```python
from build123d import *

# Parameters (mm, degrees)
F1_DEPTH = 10
F0_R     = 5
F2_DEPTH = 5
F0_W     = 12.0738212518
F0_H     = 31.9068175741
F3_DEPTH = 12.5
F4_R     = 5
F5_SIZE2 = 5
F5_SIZE  = 10
F7_DEPTH = 25
F8_W     = 7.5
F8_H     = 27.4257330972
F9_DEPTH = 15


with BuildPart() as f1:
    # F0 (on Front) → F1 (new body, symmetric)
    with BuildSketch(Plane.XZ):
        with BuildLine():
            Line((-21.1634319276, -26.7058201134), (-21.1634319276, -41.4115685539))
            ThreePointArc((-21.1634319276, -41.4115685539), (-10.6175206449, -34.455488704), (1.9829672237, -33.5438982608))
            Line((1.9829672237, -33.5438982608), (3.4650283433, -26.7058201134))
            Line((3.4650283433, -26.7058201134), (-8.6087929085, -26.7058201134))
            Line((-8.6087929085, -26.7058201134), (-21.1634319276, -26.7058201134))
        make_face()
    extrude(amount=F1_DEPTH, both=True)

    # F0 (on Front) → F2 (join, symmetric)
    with BuildSketch(Plane.XZ):
        with BuildLine():
            Line((-21.1634319276, -41.4115685539), (-21.1634319276, -53.1254634261))
            Line((-21.1634319276, -53.1254634261), (-19.8923903583, -53.1254634261))
            Line((-19.8923903583, -53.1254634261), (-11.2321363204, -53.1254634261))
            ThreePointArc((-11.2321363204, -53.1254634261), (-2.5718822826, -68.1254634261), (6.0883717553, -53.1254634261))
            Line((6.0883717553, -53.1254634261), (14.7486257931, -53.1254634261))
            Line((14.7486257931, -53.1254634261), (16.0196673624, -53.1254634261))
            Line((16.0196673624, -53.1254634261), (16.0196673624, -41.4115685539))
            ThreePointArc((16.0196673624, -41.4115685539), (9.6516199724, -36.3175292593), (1.9829672237, -33.5438982608))
            ThreePointArc((1.9829672237, -33.5438982608), (-10.6175206449, -34.455488704), (-21.1634319276, -41.4115685539))
        make_face()
        with Locations((-2.5718822826, -58.1254634261)):
            Circle(F0_R, mode=Mode.SUBTRACT)
        with BuildLine():
            Line((3.4650283433, -26.7058201134), (1.9829672237, -33.5438982608))
            ThreePointArc((1.9829672237, -33.5438982608), (9.6516199724, -36.3175292593), (16.0196673624, -41.4115685539))
            Line((16.0196673624, -41.4115685539), (16.0196673624, -26.7058201134))
            Line((16.0196673624, -26.7058201134), (3.4650283433, -26.7058201134))
        make_face()
    extrude(amount=F2_DEPTH, both=True)

    # F0 (on Front) → F3 (join, symmetric)
    with BuildSketch(Plane.XZ):
        with Locations((-2.5718822826, -10.7524113264)):
            Rectangle(F0_W, F0_H)
        Polygon((-4.447942134, 28.565781191), (-8.6087929085, 5.2009974606), (3.4650283433, 5.2009974606), (7.2547487569, 26.4817409097), align=None)
        Polygon((6.1142202467, 42.9687313735), (-4.447942134, 28.565781191), (7.2547487569, 26.4817409097), (16.6688518649, 39.3191555594), align=None)
    extrude(amount=F3_DEPTH, both=True)

    # F4
    f4_edges = [f1.edges().sort_by_distance(p)[0] for p in [
        (-8.608793, 0, 5.200997),
        (-4.447942, 0, 28.565781),
    ]]
    fillet(f4_edges, radius=F4_R)

    # F5
    f5_edges = [f1.edges().sort_by_distance(p)[0] for p in [
        (6.11422, 0, 42.968731),
    ]]
    f5_side = f1.faces().sort_by_distance((1.176582, 0, 36.235587))[0]
    chamfer(f5_edges, length=F5_SIZE, length2=F5_SIZE2, reference=f5_side)

    # F6 (on face) → F7 (cut)
    with BuildSketch(Plane(origin=(-15.3979489719, 0, 25.4772253764), x_dir=(0.8558343717, 0, 0.5172499669), z_dir=(-0.5172499669, 0, 0.8558343717))):
        with BuildLine():
            Line((30.657387603, 12.5), (30.657387603, 4.6880120664))
            ThreePointArc((30.657387603, 4.6880120664), (32.4777582205, 0), (30.657387603, -4.6880120664))
            Line((30.657387603, -4.6880120664), (30.657387603, -12.5))
            Line((30.657387603, -12.5), (39.1792431474, -12.5))
            Line((39.1792431474, -12.5), (39.1792431474, 12.5))
            Line((39.1792431474, 12.5), (30.657387603, 12.5))
        make_face()
        with BuildLine():
            Line((21.6556563973, 12.5), (21.6556563973, 9.3958744477))
            ThreePointArc((21.6556563973, 9.3958744477), (22.5944314954, 2.8906144363), (28.1230778906, 6.445016712))
            ThreePointArc((28.1230778906, 6.445016712), (29.4889605189, 5.7089196767), (30.657387603, 4.6880120664))
            Line((30.657387603, 4.6880120664), (30.657387603, 12.5))
            Line((30.657387603, 12.5), (21.6556563973, 12.5))
        make_face()
        with BuildLine():
            Line((30.657387603, -12.5), (30.657387603, -4.6880120664))
            ThreePointArc((30.657387603, -4.6880120664), (29.4889605189, -5.7089196767), (28.1230778906, -6.445016712))
            ThreePointArc((28.1230778906, -6.445016712), (22.5944314954, -2.8906144363), (21.6556563973, -9.3958744477))
            Line((21.6556563973, -9.3958744477), (21.6556563973, -12.5))
            Line((21.6556563973, -12.5), (30.657387603, -12.5))
        make_face()
    extrude(amount=-F7_DEPTH, mode=Mode.SUBTRACT)

    # F8 (on face) → F9 (cut)
    with BuildSketch(Plane(origin=(-21.1634319276, 0, 0), x_dir=(0, -1, 0), z_dir=(-1, 0, 0))):
        with Locations((0, -39.4125968775)):
            Rectangle(F8_W, F8_H)
    extrude(amount=-F9_DEPTH, mode=Mode.SUBTRACT)


solid = f1.part
```
Read the model definition and answer for the solid it produces. Units are mm, in the model's axes. A direction names the side the tool comes from. Coordinates: 2 decimals unless noted, no trailing zeros. Write each loop counter-clockwise with the first axis right and the second up, starting at its lowest first coordinate (ties: lowest second). Pieces come first, ordered by that corner, then holes. Notation, with made-up numbers: (19.5, 44) -> (63.5, 44) arc R3 cw to (63.5, 49) -> close; hole circle Ø11 at (-25.75, -3.5). An arc over 180 degrees is marked (long way). Return JSON: item names as keys, results as strings.
1. A cutting plane is placed at C-C (z = -29.5). Determine the outline of the cut face in (x, y).
Found:
{"outline": "(-21.16, -10) -> (2.86, -10) -> (2.86, -5) -> (16.02, -5) -> (16.02, 5) -> (2.86, 5) -> (2.86, 10) -> (-21.16, 10) -> (-21.16, 3.75) -> (-6.16, 3.75) -> (-6.16, -3.75) -> (-21.16, -3.75) -> close"}
2. A cutting plane is placed at D-D (x = -19). Determine the outline of the cut face in (y, z).
Found:
{"outline": "(-10, -39.28) -> (-5, -39.28) -> (-5, -53.13) -> (-3.75, -53.13) -> (-3.75, -26.71) -> (-10, -26.71) -> close; (3.75, -53.13) -> (5, -53.13) -> (5, -39.28) -> (10, -39.28) -> (10, -26.71) -> (3.75, -26.71) -> close"}
3. Determine the mould class of faces 1 (the face through (-12, 10, -31)), 2 (the face through (6.607, 2.937, 32.559)), 3 (the face through (-21.163, -6, -37)), 4 (the face through (-12, -10, -31)) for opening direction Y: pulls with the +Y half, pulls with the -Y half, needs draft (parallel to the pull), parting line crosses it, or undercut.
Found:
{"face 1": "pulls with the +Y half", "face 2": "undercut", "face 3": "needs draft", "face 4": "pulls with the -Y half"}
4. A cutting plane is placed at A-A (x = -14). Determine the outline of the cut face in (y, z).
Found:
{"outline": "(-10, -35.89) -> (-5, -35.89) -> (-5, -53.13) -> (-3.75, -53.13) -> (-3.75, -26.71) -> (-10, -26.71) -> close; (3.75, -53.13) -> (5, -53.13) -> (5, -35.89) -> (10, -35.89) -> (10, -26.71) -> (3.75, -26.71) -> close"}
5. Find the intervals of material crossed by line 1 along Y through (x, z) = (-12, -41); line 2 along Y through (x, z) = (7, 29.5); line 3 along X through (y, z) = (-3.5, -48), in increasing order. Write a range as from..to.
Found:
{"line 1": "-5..-3.75, 3.75..5", "line 2": "-12.5..-8.99, -3.9..3.9, 8.99..12.5", "line 3": "-6.16..16.02"}
6. A tool of negligible diameter and unlimited length cuts with its end or side. For faces 5 (the face through (-10.787, -7.535, -34.514)), 6 (the face through (-9, 0, -53.125)), 7 (the face through (5.72, -10.93, 32.4)), 8 (the face through (2.714, -7.535, -30.173)), 9 (the face through (-8.609, 0, -11)), from which of +Z, -Z, +X, -X, +Y, -Y can it reach the whole face along a straight path? Write none if from no direction.
Found:
{"face 5": "-Z, -Y", "face 6": "-X", "face 7": "+Z, +X, -Y", "face 8": "-Z, +X, -Y", "face 9": "+Z, -X, +Y, -Y"}
7. A cutting plane is placed at B-B (y = 7.5). Determine the outline of the cut face in (x, z).
Found:
{"outline": "(-21.16, -41.41) arc R25 cw to (1.98, -33.54) -> (3.47, -26.71) -> (3.47, 5.2) -> (7.25, 26.48) -> (7.61, 26.96) -> (2.11, 36.06) -> (0.2, 34.9) -> (-3.76, 29.5) arc R5 ccw to (-4.65, 27.42) -> (-8.53, 5.64) arc R5 ccw to (-8.61, 4.76) -> (-8.61, -26.71) -> (-21.16, -26.71) -> close"}
8. Each of these flat-tipped pins is pushed along its axis until it touches: P1, Ø12, axis at x = -5.5, y = -2, coming from the +Z side; P2, Ø7, axis at x = -15, y = 5.5, coming from the +Z side; P3, Ø4.5, axis at x = -10.5, z = -39.5, coming from the -Y side. Where does it stop, or does it pass through?
Found:
{"P1": "z = 35.09", "P2": "z = -26.71", "P3": "y = -5"}
